Build history of the part. All positions in model axes, mm. A direction names the side the tool comes from. Round coordinates to 2 decimals unless told otherwise and drop trailing zeros. Loops run counter-clockwise (first coordinate to the right, second up) from the corner with the lowest first, then second, coordinate; pieces in that order, holes last. Notation, with made-up numbers: (13.25, -17) - (49.25, -17) arc R24 cw to (49.25, 17) - close; hole circle Ø1 at (40.25, 38). An arc over 180 degrees is marked (long way). Put each result on its own line as item: value. Start each with the question number.
from build123d import *

# Parameters (mm, degrees)
F0_W     = 14.75
F0_H     = 9
F1_DEPTH = 4
F2_R     = 2.4
F3_D     = 1.9


with BuildPart() as f1:
    # F0 (on Front) → F1 (new body)
    with BuildSketch(Plane.XZ):
        Polygon((-24.125, 46.5), (-29.5, 46.5), (-29.5, -4), (29.5, -4), (29.5, 46.5), (-3.375, 46.5), (-3.375, 58.5), (-24.125, 58.5), align=None)
        Polygon((-2, 42.5), (-2, 0), (-25.5, 0), (-25.5, 19.25), (-25.2, 19.25), (-25.2, 23.25), (-25.5, 23.25), (-25.5, 42.5), align=None, mode=Mode.SUBTRACT)
        Polygon((25.5, 0), (2, 0), (2, 42.5), (25.5, 42.5), (25.5, 23.25), (25.2, 23.25), (25.2, 19.25), (25.5, 19.25), align=None, mode=Mode.SUBTRACT)
        with Locations((-13.75, 51)):
            Rectangle(F0_W, F0_H, mode=Mode.SUBTRACT)
    extrude(amount=F1_DEPTH)

    # F2
    f2_edges = [f1.edges().sort_by_distance(p)[0] for p in [
        (-24.125, -2, 58.5),
        (-24.125, -2, 46.5),
        (-29.5, -2, 46.5),
        (-3.375, -2, 58.5),
        (29.5, -2, 46.5),
        (-3.375, -2, 46.5),
        (29.5, -2, -4),
        (-29.5, -2, -4),
    ]]
    fillet(f2_edges, radius=F2_R)

    # F3 (through all)
    with Locations(Plane(origin=(0, 0, 0), x_dir=(1, 0, 0), z_dir=(0, 1, 0))):
        with Locations((-13.75, 2), (13.75, 2), (-13.75, -44.5), (13.75, -44.5)):
            Hole(F3_D / 2)


solid = f1.part
1) Slice it at A-A, the plane x = -13.75. Write the cut outline in (y, z), and give its area (3 significant figures).
2) Slice it at C-C, the plane x = 19.5. Write the cut outline in (y, z).
3) Slice it at B-B, the plane z = 10.5. Write the cut outline in (x, y).
4) Drill centre lines: line 1 (Z direction, x = 13.75, y = -1.2); line 2 (X direction, y = -1, z = 6); line 3 (Z direction, x = -13.75, y = -1.05). Where is each one in solid material? Low to high. Write a range as [from, to].
5) Which spindle directions (+Z, -Z, +X, -X, +Y, -Y) get a long thin tool onto all of the face, cutting with end or side? Do faces 1 (the face through (25.5, -2, 10)), 2 (the face through (-28.816, -2.028, -3.278)), 3 (the face through (13, -2, 46.5)). Say none if no direction does.
6) Pull direction X, two halves, no side cores. Call faces 4 (the face through (-25.5, -2, 9)), 5 (the face through (-24.125, -2, 53)), 6 (the face through (0, -2, -4)): pulls with the +X half, pulls with the -X half, needs draft (parallel to the pull), parting line crosses it, or undercut.
7) Slice it at D-D, the plane y = -2.7. State how many separate pieces and enclosed holes the cut face has, and give its area (3 significant figures).
Taken from the geometry:
1. outline: (-4, -4) - (0, -4) - (0, -2.95) - (-4, -2.95) - close; (-4, -1.05) - (0, -1.05) - (0, 0) - (-4, 0) - close; (-4, 42.5) - (0, 42.5) - (0, 43.55) - (-4, 43.55) - close; (-4, 45.45) - (0, 45.45) - (0, 46.5) - (-4, 46.5) - close; (-4, 55.5) - (0, 55.5) - (0, 58.5) - (-4, 58.5) - close
1. area: 28.8 mm2
2. outline: (-4, -4) - (0, -4) - (0, 0) - (-4, 0) - close; (-4, 42.5) - (0, 42.5) - (0, 46.5) - (-4, 46.5) - close
3. outline: (-29.5, -4) - (-25.5, -4) - (-25.5, 0) - (-29.5, 0) - close; (-2, -4) - (2, -4) - (2, 0) - (-2, 0) - close; (25.5, -4) - (29.5, -4) - (29.5, 0) - (25.5, 0) - close
4. line 1: z = [-4, -2.95], [-1.05, 0], [42.5, 43.55], [45.45, 46.5]
4. line 2: x = [-29.5, -25.5], [-2, 2], [25.5, 29.5]
4. line 3: z = [-4, -2.95], [-1.05, 0], [42.5, 43.55], [45.45, 46.5], [55.5, 58.5]
5. face 1: +Y, -Y
5. face 2: -Z, -X, +Y, -Y
5. face 3: +Z, +X, +Y, -Y
6. face 4: undercut
6. face 5: pulls with the -X half
6. face 6: needs draft
7. separate pieces: 1
7. enclosed holes: 7
7. area: 1,080 mm2
